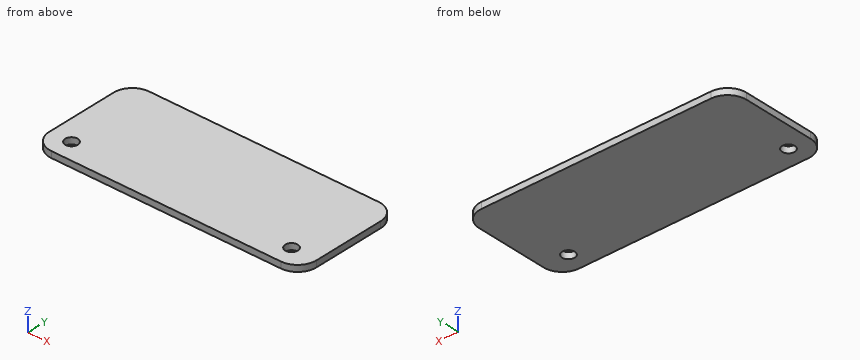
Autodesk Inventor part; units mm, degrees
ref_plane "YZ Plane" through (0, 0, 0) normal (1, 0, 0) x (0, 1, 0)
ref_plane "XZ Plane" through (0, 0, 0) normal (0, 1, 0) x (-1, 0, 0)
ref_plane "XY Plane" through (0, 0, 0) normal (0, 0, 1) x (1, 0, 0)
sketch "Sketch1" plane through (0, 0, 0) normal (0, 0, 1) x (1, 0, 0)
  line L0 (-35.8578, -17.234) -> (37.1422, -17.234)
  arc A0 (37.1422, -17.234) -> (43.1422, -11.234) centre (37.1422, -11.234) ccw
  line L1 (43.1422, -11.234) -> (43.1422, 11.766)
  arc A1 (43.1422, 11.766) -> (37.1422, 17.766) centre (37.1422, 11.766) ccw
  line L2 (37.1422, 17.766) -> (-35.8578, 17.766)
  arc A2 (-35.8578, 17.766) -> (-41.8578, 11.766) centre (-35.8578, 11.766) ccw
  line L3 (-41.8578, 11.766) -> (-41.8578, -11.234)
  arc A3 (-41.8578, -11.234) -> (-35.8578, -17.234) centre (-35.8578, -11.234) ccw
  arc A4 (41.1422, 12.766) -> (38.1422, 15.766) centre (38.1422, 12.766) ccw
  line L4 (41.1422, 12.766) -> (41.1422, -12.234)
  arc A5 (38.1422, -15.234) -> (41.1422, -12.234) centre (38.1422, -12.234) ccw
  line L5 (38.1422, -15.234) -> (-36.8578, -15.234)
  arc A6 (-39.8578, -12.234) -> (-36.8578, -15.234) centre (-36.8578, -12.234) ccw
  line L6 (-39.8578, -12.234) -> (-39.8578, 12.766)
  arc A7 (-36.8578, 15.766) -> (-39.8578, 12.766) centre (-36.8578, 12.766) ccw
  line L7 (-36.8578, 15.766) -> (38.1422, 15.766)
  point P0 (0, 0)
  point P1 (0.6422, 0.266)
extrude "Extrusion1" add sketch "Sketch1" along normal blind 2 contours A3 L3 A2 L2 A1 L1 A0 L0 | L4 A5 L5 A6 L6 A7 L7 A4
sketch "Sketch2" plane through (0, 0, 2) normal (0, 0, 1) x (1, 0, 0)
  line L0 (0, 0) -> (-35, 0)
  line L1 (-35, 0) -> (-35, -11)
  line L2 (-35, -11) -> (35, -11)
  line L3 (-35, -9) -> (-35, -9)
  line L4 (-33, -11) -> (-33, -11)
  line L5 (-35, -13) -> (-35, -13)
  line L6 (-37, -11) -> (-37, -11)
  line L7 (-37, -9) -> (-33, -13) construction
  line L8 (-33, -9) -> (-37, -13) construction
  line L9 (35, -9) -> (35, -9)
  line L10 (37, -11) -> (37, -11)
  line L11 (35, -13) -> (35, -13)
  line L12 (33, -11) -> (33, -11)
  line L13 (33, -9) -> (37, -13) construction
  line L14 (37, -9) -> (33, -13) construction
  arc A0 (35, -9) -> (33, -11) centre (35, -11) ccw
  arc A1 (37, -11) -> (35, -9) centre (35, -11) ccw
  arc A2 (33, -11) -> (35, -13) centre (35, -11) ccw
  arc A3 (35, -13) -> (37, -11) centre (35, -11) ccw
  arc A4 (-33, -11) -> (-35, -9) centre (-35, -11) ccw
  arc A5 (-35, -13) -> (-33, -11) centre (-35, -11) ccw
  arc A6 (-37, -11) -> (-35, -13) centre (-35, -11) ccw
  arc A7 (-35, -9) -> (-37, -11) centre (-35, -11) ccw
  dimension "d2" = 35
  dimension "d3" = 11
  dimension "d4" = 70
  dimension "d5" = 4
  dimension "d6" = 4
  dimension "d7" = 4
  dimension "d8" = 4
  dimension "d9" = 2
extrude "Extrusion2" cut sketch "Sketch2" against normal blind 2
properties part number "CASE_1"
Design review of the part built by this model. Coordinates are the model's own, in mm. Coordinates: 2 decimals unless noted, no trailing zeros. Write each loop counter-clockwise with the first axis right and the second up, starting at its lowest first coordinate (ties: lowest second). Pieces come first, ordered by that corner, then holes. Notation, with made-up numbers: (-20.5, 38.25) - (5.5, 38.25) arc R32 ccw to (5.5, 72.25) - close; hole circle Ø5 at (58.25, -15). An arc over 180 degrees is marked (long way). One line per item, written item: value.
1) Add section C-C (x = 36). State the section outline as (y, z) points.
Answer sheet:
outline: (-17.23, 0) - (-12.73, 0) - (-12.73, 2) - (-17.23, 2) - close; (-9.27, 0) - (17.77, 0) - (17.77, 2) - (-9.27, 2) - close
2) To check wall thickness, follow probe 1 along X at (y, z) = (-11, 1.05); probe 2 along Y at (x, z) = (-35, 1.2); probe 3 along X at (y, z) = (12.5, 0.45). State the ranges of each line that lie inside material, in increasing order.
Answer sheet:
probe 1: x = -41.86 to -37, -33 to 33, 37 to 43.14
probe 2: y = -17.23 to -13, -9 to 17.77
probe 3: x = -41.81 to 43.1
3) Add section B-B (x = -35). State the section outline as (y, z) points.
Answer sheet:
outline: (-17.23, 0) - (-13, 0) - (-13, 2) - (-17.23, 2) - close; (-9, 0) - (17.77, 0) - (17.77, 2) - (-9, 2) - close
4) Add section A-A (z = 1.2). State the section outline as (x, y) points, plus the area to 3 significant figures.
Answer sheet:
outline: (-41.86, -11.23) arc R6 ccw to (-35.86, -17.23) - (37.14, -17.23) arc R6 ccw to (43.14, -11.23) - (43.14, 11.77) arc R6 ccw to (37.14, 17.77) - (-35.86, 17.77) arc R6 ccw to (-41.86, 11.77) - close; hole circle Ø4 at (-35, -11); hole circle Ø4 at (35, -11)
area: 2,920 mm2
